Design review of the part shown in the three views and the two pictorial views. Dimensions are in mm from the part's minimum x, y and z. A direction names the side the tool comes from. Coordinates: 2 decimals unless noted, no trailing zeros. Write each loop counter-clockwise with the first axis right and the second up, starting at its lowest first coordinate (ties: lowest second). Pieces come first, ordered by that corner, then holes. Notation, with made-up numbers: M 43,71 L 96,71 A13 ccw 96,90 Z; hole C 21,-38.5 d2. An arc over 180 degrees is marked long. Answer as a JSON object with one key per item and string values.
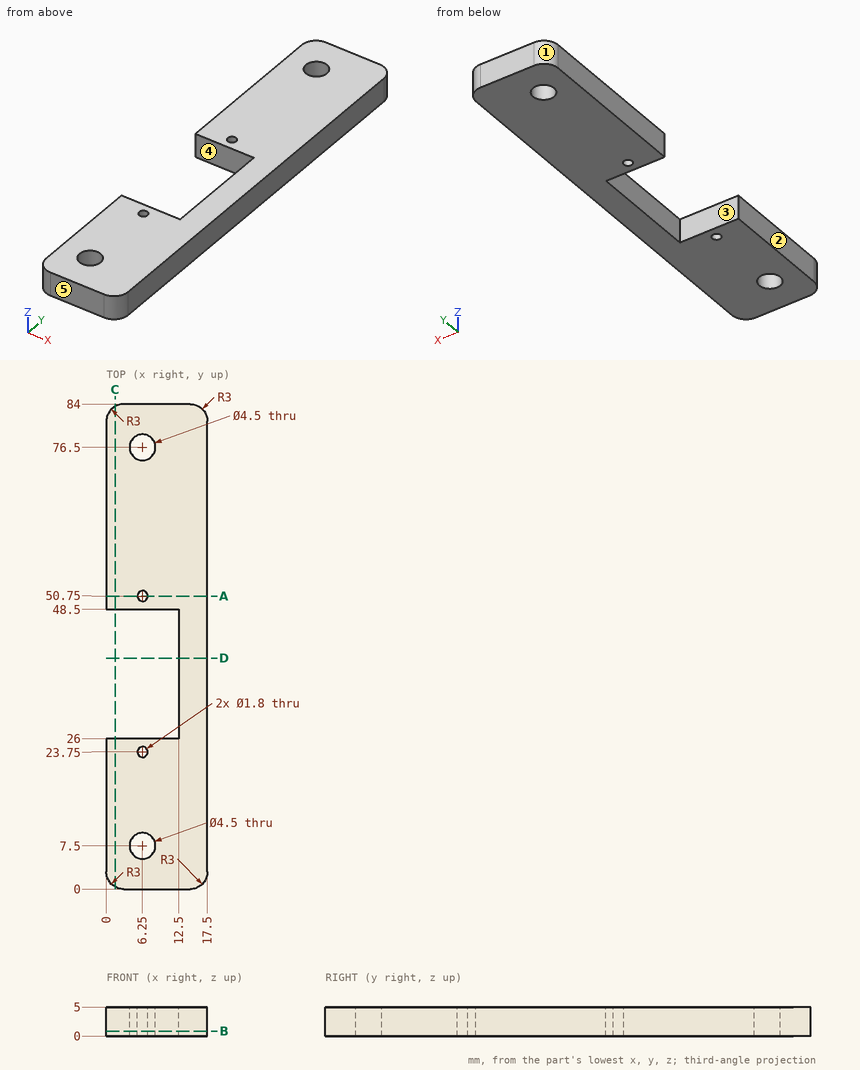
(1) Add section D-D on y = 40. Give the boundary of the cut face in (x, z).
Results list:
{"outline": "M 12.5,0 L 17.5,0 L 17.5,5 L 12.5,5 Z"}
(2) Add section B-B on z = 0.85. Give the boundary of the cut face in (x, y).
Results list:
{"outline": "M 0,3 A3 ccw 3,0 L 14.5,0 A3 ccw 17.5,3 L 17.5,81 A3 ccw 14.5,84 L 3,84 A3 ccw 0,81 L 0,48.5 L 12.5,48.5 L 12.5,26 L 0,26 Z; hole C 6.25,7.5 d4.5; hole C 6.25,76.5 d4.5; hole C 6.25,23.75 d1.8; hole C 6.25,50.75 d1.8"}
(3) Add section A-A on y = 50.75. Give the boundary of the cut face in (x, z), and give its area (3 significant figures).
Results list:
{"outline": "M 0,0 L 5.35,0 L 5.35,5 L 0,5 Z; M 7.15,0 L 17.5,0 L 17.5,5 L 7.15,5 Z", "area": "78.5 mm²"}
(4) For pin 1 Ø2.5 at (x, y) = (6.25, 76.5) entering from +Z; pin 2 Ø1 at (y, z) = (32.5, 2.5) entering from -X, all flat-tipped, find the tip position at first contact; note any pin that passes through.
Results list:
{"pin 1": "through", "pin 2": "x = 12.5"}
(5) Draft analysis for pull direction Y (two halves, no side actions). For the marked faces 1, 2 and 3, state which applies: released by +Y, released by -Y, zero draft, split by the parting line, or undercut.
Results list:
{"face 1": "released by +Y", "face 2": "zero draft", "face 3": "undercut"}
(6) Wall thickness on line 1 along Y through (x, z) = (6.25, 1.7); line 2 along Y through (x, z) = (9.75, 1.5); line 3 along X through (y, z) = (50.75, 1.7): over which ranges is each line inside the solid? List them lowest first. Write a range as from..to.
Results list:
{"line 1": "0..5.25, 9.75..22.85, 24.65..26, 48.5..49.85, 51.65..74.25, 78.75..84", "line 2": "0..26, 48.5..84", "line 3": "0..5.35, 7.15..17.5"}
(7) For the marked faces 4 and 5, list the 3-axis set-ups (+Z, -Z, +X, -X, +Y, -Y) from which the entire face can be reached by the end or side of a thin tool; tool diameter is ignored.
Results list:
{"face 4": "+Z, -Z, -X", "face 5": "+Z, -Z, +X, -X, -Y"}
(8) Add section C-C on x = 1.5. Give the boundary of the cut face in (y, z), and give its area (3 significant figures).
Results list:
{"outline": "M 0.4,0 L 26,0 L 26,5 L 0.4,5 Z; M 48.5,0 L 83.6,0 L 83.6,5 L 48.5,5 Z", "area": "303 mm²"}
